Check sheet for the modelled part. Datum: model origin and axes. Units: mm. A direction names the side the tool comes from. Give positions to 0.01 mm unless a question says otherwise; leave off trailing zeros. Loops run counter-clockwise (first coordinate to the right, second up) from the corner with the lowest first, then second, coordinate; pieces in that order, holes last. Notation, with made-up numbers: (89.5, 26.5) - (134.5, 26.5) arc R23 ccw to (134.5, 62.5) - close; hole circle Ø2 at (-15.75, 69). An arc over 180 degrees is marked (long way). Use CSV: the item, a comma, the result in double quotes.
from build123d import *


with BuildPart() as part:
    # Sketch1 → Revolve1 (revolve)
    with BuildSketch(Plane.XY):
        with BuildLine():
            Line((0, 0), (20, 0))
            Line((20, 0), (20, 80))
            Line((20, 80), (30, 80))
            Line((30, 80), (30, 85))
            Line((30, 85), (20, 85))
            Line((20, 85), (20, 95.717967697))
            ThreePointArc((20, 95.717967697), (40, 130.358983849), (20, 165))
            Line((20, 165), (0, 165))
            Line((0, 165), (0, 0))
        make_face()
    revolve(axis=Axis((0, 0, 0), (0, 1, 0)))


solid = part.part
1. Scan lines: line 1 along Y through (x, z) = (21, -19); line 2 along Y through (x, z) = (-12.5, 18.5); line 3 along X through (y, z) = (144, 3.5). Record each from-to range of solid material in increasing order.
Completed:
line 1,"y = 80 to 85, 102.11 to 158.61"
line 2,"y = 80 to 85, 97.17 to 163.55"
line 3,"x = -37.44 to 37.44"
2. Release check for a two-part mould opening along Y. For faces 3 (the face through (0, 165, 0)), 4 (the face through (-4.336, 90.434, 19.524)), 5 (the face through (-6, 80, 20)), 6 (the face through (6, 85, 20)) record: released by +Y, released by -Y, zero draft, split by the parting line, or undercut.
Completed:
face 3,"released by +Y"
face 4,"undercut"
face 5,"released by -Y"
face 6,"undercut"
3. Sectioned sample at B-B, the plane x = 0. Record the boundary of the cut face in (y, z).
Completed:
outline,"(0, -20) - (80, -20) - (80, -30) - (85, -30) - (85, -20) - (95.72, -20) arc R40 ccw to (165, -20) - (165, 20) arc R40 ccw to (95.72, 20) - (85, 20) - (85, 30) - (80, 30) - (80, 20) - (0, 20) - close"
4. Sectioned sample at C-C, the plane z = -26. Record the boundary of the cut face in (x, y), and give its area (3 significant figures).
Completed:
outline,"circle Ø60.79 at (0, 130.36); (-14.97, 80) - (14.97, 80) - (14.97, 85) - (-14.97, 85) - close"
area,"3,050 mm²"
5. Set-up check for faces 1 (the face through (-4.336, 40.56, 19.524)), 2 (the face through (0, 0, 0)): record each of +Z, -Z, +X, -X, +Y, -Y from which the full face is reachable in a straight line by a thin tool's end or side.
Completed:
face 1,"-Y"
face 2,"+Z, -Z, +X, -X, -Y"
6. Sectioned sample at A-A, the plane z = 0. Record the boundary of the cut face in (x, y), and give its area (3 significant figures).
Completed:
outline,"(-30, 80) - (-20, 80) - (-20, 0) - (20, 0) - (20, 80) - (30, 80) - (30, 85) - (20, 85) - (20, 95.72) arc R40 ccw to (20, 165) - (-20, 165) arc R40 ccw to (-20, 95.72) - (-20, 85) - (-30, 85) - close"
area,"8,670 mm²"
7. Sectioned sample at D-D, the plane y = 37. Record the boundary of the cut face in (x, z).
Completed:
outline,"circle Ø40 at (0, 0)"
8. Go/stop test with flat-tipped pins: pin 1 Ø5 at (y, z) = (128, 32) entering from +X; pin 2 Ø4 at (x, z) = (22.5, 16.5) entering from -Y; pin 3 Ø4 at (x, y) = (-16, 73.5) entering from -Z. Record where each tip stops, or that it passes through.
Completed:
pin 1,"stops at x = 26.92"
pin 2,"stops at y = 80"
pin 3,"stops at z = -14.28"
